CAD build for the part. Positions are in the model's coordinates, mm. A direction names the side the tool comes from. Give positions to 0.01 mm unless a question says otherwise; leave off trailing zeros. Write each loop counter-clockwise with the first axis right and the second up, starting at its lowest first coordinate (ties: lowest second). Pieces come first, ordered by that corner, then holes. Notation, with made-up numbers: (43.25, 88.5) -> (50.25, 88.5) arc R18 cw to (50.25, 116.5) -> close; hole circle Ø4 at (-26.5, 47). An arc over 180 degrees is marked (long way). Answer in a Markdown table with one row per item. Add a question column.
```python
from build123d import *

# Parameters (mm, degrees)
SKETCH008_W          = 9.417664
SKETCH008_H          = 8.015827
PAD_DEPTH            = 6
SKETCH007_W          = 17.214357
SKETCH007_H          = 23
PAD001_DEPTH         = 4
SKETCH_W             = 41
SKETCH_H             = 23
PAD002_DEPTH         = 3
SKETCH009_W          = 6
SKETCH009_H          = 8
PAD003_DEPTH         = 4
POCKET_DEPTH         = 1.5
POCKET001_DEPTH      = 5
POCKET002_DEPTH      = 5
POCKET003_DEPTH      = 5
POCKET004_DEPTH      = 5
SKETCH004_R          = 2.5
POCKET005_DEPTH      = 5
SKETCH010_W          = 41
SKETCH010_H          = 2
SKETCH010_W_2        = 31.58
POCKET006_DEPTH      = 5
SKETCH013_W          = 2
SKETCH013_H          = 2.18
POCKET007_DEPTH      = 10
SKETCH014_W          = 2.7
SKETCH014_H          = 5
POCKET008_DEPTH      = 10
POCKET008_DEPTH_BACK = 10
SKETCH015_W          = 1
SKETCH015_H          = 2.1
POCKET009_DEPTH      = 8.05
SKETCH012_R          = 0.8
POCKET010_DEPTH      = 8
SKETCH016_R          = 0.5
POCKET011_DEPTH      = 1
SKETCH017_W          = 38
SKETCH017_H          = 20
SKETCH017_W_2        = 35
SKETCH017_H_2        = 17
POCKET012_DEPTH      = 0.5


with BuildPart() as part:
    # Sketch008 → Pad (new body)
    with BuildSketch(Plane.XY):
        with Locations((36.336342, 4.0079135)):
            Rectangle(SKETCH008_W, SKETCH008_H)
    extrude(amount=PAD_DEPTH)

    # Sketch007 → Pad001 (join)
    with BuildSketch(Plane.XY):
        with Locations((32.3928215, 11.5)):
            Rectangle(SKETCH007_W, SKETCH007_H)
    extrude(amount=PAD001_DEPTH)

    # Sketch → Pad002 (join)
    with BuildSketch(Plane.XY):
        with Locations((20.5, 11.5)):
            Rectangle(SKETCH_W, SKETCH_H)
    extrude(amount=PAD002_DEPTH)

    # Sketch009 → Pad003 (join)
    with BuildSketch(Plane.XY):
        with Locations((3.029941472, 11.1135029832)):
            Rectangle(SKETCH009_W, SKETCH009_H)
    extrude(amount=PAD003_DEPTH)

    # Sketch003 → Pocket (cut)
    with BuildSketch(Plane.XY):
        with BuildLine():
            Line((23.975689, 13.0540965715), (26.8011965151, 13.0540965715))
            ThreePointArc((26.8011965151, 13.0540965715), (27.3647082361, 13.2875107689), (27.5981224335, 13.8510224899))
            Line((27.5981224335, 13.8510224899), (27.5981224335, 14.526678))
            Line((27.5981224335, 14.526678), (30.5981224335, 14.526678))
            Line((30.5981224335, 14.526678), (30.5981224335, 13.2924514667))
            ThreePointArc((27.3597675383, 10.0540965715), (29.6496302446, 11.0025887604), (30.5981224335, 13.2924514667))
            Line((27.3597675383, 10.0540965715), (23.975689, 10.0540965715))
            Line((23.975689, 10.0540965715), (23.975689, 13.0540965715))
        make_face()
    extrude(amount=POCKET_DEPTH, mode=Mode.SUBTRACT)

    # Sketch001 → Pocket001 (cut)
    with BuildSketch(Plane.XY):
        with BuildLine():
            ThreePointArc((6.1032483008, 13.3387395872), (4.7679879703, 11.5907435275), (5.8459964121, 9.6733734082))
            Line((5.8459964121, 9.6733734082), (11.4677626675, 6.8598227367))
            ThreePointArc((11.4677626675, 6.8598227367), (14.6035600083, 5.8212239037), (17.794301339, 6.6762573881))
            Line((17.794301339, 6.6762573881), (23.3375945955, 9.6414256942))
            ThreePointArc((23.3375945955, 9.6414256942), (24.7768585387, 11.4984422833), (23.4574990247, 13.4424797786))
            Line((23.4574990247, 13.4424797786), (17.8173054197, 16.4670815869))
            ThreePointArc((17.8173054197, 16.4670815869), (14.6646196223, 17.3378254465), (11.5461110533, 16.3516576556))
            Line((11.5461110533, 16.3516576556), (6.1032483008, 13.3387395872))
        make_face()
    extrude(amount=POCKET001_DEPTH, mode=Mode.SUBTRACT)

    # Sketch006 → Pocket002 (cut)
    with BuildSketch(Plane.XY.offset(1.5)):
        with BuildLine():
            ThreePointArc((30.093781, 6.846887), (27.593781, 9.346887), (25.093781, 6.846887))
            Line((25.093781, 6.846887), (25.093781, 5.346887))
            ThreePointArc((25.093781, 5.346887), (27.593781, 2.846887), (30.093781, 5.346887))
            Line((30.093781, 6.846887), (30.093781, 5.346887))
        make_face()
    extrude(amount=POCKET002_DEPTH, mode=Mode.SUBTRACT)

    # Sketch005 → Pocket003 (cut)
    with BuildSketch(Plane.XY.offset(1.5)):
        with BuildLine():
            ThreePointArc((31.548714, 10.251081), (34.048714, 7.751081), (36.548714, 10.251081))
            Line((36.548714, 10.251081), (36.548714, 17.751081))
            ThreePointArc((36.548714, 17.751081), (34.048714, 20.251081), (31.548714, 17.751081))
            Line((31.548714, 10.251081), (31.548714, 17.751081))
        make_face()
    extrude(amount=POCKET003_DEPTH, mode=Mode.SUBTRACT)

    # Sketch002 → Pocket004 (cut)
    with BuildSketch(Plane.XY):
        with BuildLine():
            ThreePointArc((28.798038, 18.6125900268), (26.1467217956, 15.9612738224), (28.798038, 13.3099576181))
            Line((28.798038, 13.309957618), (33.4782685239, 13.309957618))
            ThreePointArc((33.4782685239, 13.3099576181), (36.1295847282, 15.9612738224), (33.4782685239, 18.6125900268))
            Line((28.798038, 18.6125900268), (33.4782685239, 18.6125900268))
        make_face()
    extrude(amount=POCKET004_DEPTH, mode=Mode.SUBTRACT)

    # Sketch004 → Pocket005 (cut)
    with BuildSketch(Plane.XY):
        with Locations((34, 10.25)):
            Circle(SKETCH004_R)
    extrude(amount=POCKET005_DEPTH, mode=Mode.SUBTRACT)

    # Sketch010 → Pocket006 (cut)
    with BuildSketch(Plane.XY.offset(1.8)):
        with Locations((20.5, 22)):
            Rectangle(SKETCH010_W, SKETCH010_H)
        with Locations((15.79, 1)):
            Rectangle(SKETCH010_W_2, SKETCH010_H)
    extrude(amount=POCKET006_DEPTH, mode=Mode.SUBTRACT)

    # Sketch013 → Pocket007 (cut)
    with BuildSketch(Plane.YZ.offset(31.58)):
        with Locations((1, 2.89)):
            Rectangle(SKETCH013_W, SKETCH013_H)
    extrude(amount=POCKET007_DEPTH, mode=Mode.SUBTRACT)

    # Sketch014 → Pocket008 (cut, two sides)
    with BuildSketch(Plane(origin=(0, -2.5, 0), x_dir=(1, 0, 0), z_dir=(0, -0.8660254038, 0.5))) as pocket008_sk:
        with Locations((34.35, 8.5)):
            Rectangle(SKETCH014_W, SKETCH014_H)
    extrude(amount=-POCKET008_DEPTH, mode=Mode.SUBTRACT)
    extrude(pocket008_sk.sketch, amount=POCKET008_DEPTH_BACK, mode=Mode.SUBTRACT)

    # Sketch015 → Pocket009 (cut)
    with BuildSketch(Plane.XZ):
        with Locations((38.5, 5.0085653562)):
            Rectangle(SKETCH015_W, SKETCH015_H)
    extrude(amount=-POCKET009_DEPTH, mode=Mode.SUBTRACT)

    # Sketch012 → Pocket010 (cut)
    with BuildSketch(Plane(origin=(5, 0, 0), x_dir=(0, 1, 0), z_dir=(0.9396926208, 0, -0.3420201433))):
        with Locations((11.55, 1)):
            Circle(SKETCH012_R)
    extrude(amount=-POCKET010_DEPTH, mode=Mode.SUBTRACT)

    # Sketch016 → Pocket011 (cut, symmetric)
    with BuildSketch(Plane(origin=(0, 1, 0.2), x_dir=(1, 0, 0), z_dir=(0, -0.8660254038, 0.5))):
        with Locations((27.497313, 2.982959)):
            Circle(SKETCH016_R)
    extrude(amount=POCKET011_DEPTH, both=True, mode=Mode.SUBTRACT)

    # Sketch017 → Pocket012 (cut)
    with BuildSketch(Plane.XY):
        with Locations((20.5, 11.5)):
            Rectangle(SKETCH017_W, SKETCH017_H)
        with Locations((20.5, 11.5)):
            Rectangle(SKETCH017_W_2, SKETCH017_H_2, mode=Mode.SUBTRACT)
    extrude(amount=POCKET012_DEPTH, mode=Mode.SUBTRACT)


solid = part.part
```
Item 1: Which spindle directions (+Z, -Z, +X, -X, +Y, -Y) get a long thin tool onto all of the face, cutting with end or side? Do faces 1 (the face through (20.68, 14.93, 1.48)), 2 (the face through (38.5, 5, 3.959)), 3 (the face through (25, 13.054, 1)). Say none if no direction does.
Item 2: Slice it at B-B, the plane z = 4.5. List the corners of the cut face in (x, y), then the cut area to 3 significant figures.
Item 3: Mould opens along Y. For faces 4 (the face through (40, 0, 5)), 5 (the face through (39, 4, 5)), 6 (the face through (20.53, 8.14, 1.48)) say: released by +Y, released by -Y, zero draft, split by the parting line, or undercut.
Item 4: Slice it at C-C, the plane x = 34. List the corners of the cut face in (y, z).
Item 5: Slice it at A-A, the plane x = 14. List the corners of the cut face in (y, z).
Item 6: Probe L1, parallel to X at y = 10.25, z = 1.75; L2, parallel to X at y = 16.25, z = 1; L3, parallel to Z at x = 7, y = 15.5. List the from-to ranges inside material, lowest first. Write a range as from..to.
Item 7: Slice it at D-D, the plane y = 19.5. List the corners of the cut face in (x, z).
Item 8: Drop flat-ended pins along their axis: pin 1 Ø1 at (x, z) = (31.5, 3) entering from +Y; pin 2 Ø0.8 at (x, y) = (38.5, 4) entering from +Z; pin 3 Ø1 at (y, z) = (16.5, 5.5) entering from +X; pin 4 Ø1 at (x, z) = (32.5, 5) entering from +Y. Give the stop position or say it passes through.
Answer key:
| question | item | result |
|---|---|---|
| 1 | face 1 | +Z, -Z |
| 1 | face 2 | +Z, -Y |
| 1 | face 3 | -Z |
| 2 | outline | (31.63, 0) -> (38, 0) -> (38, 8.02) -> (35.7, 8.02) -> (35.7, 1.71) -> (33, 1.71) -> (33, 7.96) arc R2.5 cw to (32.88, 8.02) -> (31.63, 8.02) -> close; (39, 0) -> (41.05, 0) -> (41.05, 8.02) -> (39, 8.02) -> close |
| 2 | area | 50.4 mm² |
| 3 | face 4 | released by -Y |
| 3 | face 5 | zero draft |
| 3 | face 6 | undercut |
| 4 | outline | (0, 0) -> (1.5, 0) -> (1.5, 0.5) -> (3, 0.5) -> (3, 0) -> (7.75, 0) -> (7.75, 1.01) -> (0, 5.48) -> (0, 3.98) -> (2, 3.98) -> (2, 1.8) -> (0, 1.8) -> close; (12.75, 0) -> (13.36, 0) -> (13.36, 1.5) -> (12.75, 1.5) -> close; (18.56, 0) -> (20, 0) -> (20, 0.5) -> (21.5, 0.5) -> (21.5, 0) -> (23, 0) -> (23, 1.8) -> (21, 1.8) -> (21, 4) -> (20.25, 4) -> (20.25, 1.5) -> (18.56, 1.5) -> close |
| 5 | outline | (0, 0) -> (1.5, 0) -> (1.5, 0.5) -> (3, 0.5) -> (3, 0) -> (5.87, 0) -> (5.87, 3) -> (2, 3) -> (2, 1.8) -> (0, 1.8) -> close; (17.29, 0) -> (20, 0) -> (20, 0.5) -> (21.5, 0.5) -> (21.5, 0) -> (23, 0) -> (23, 1.8) -> (21, 1.8) -> (21, 3) -> (17.29, 3) -> close |
| 6 | L1 | x = 0..5.16, 24.29..31.5, 36.55..41 |
| 6 | L2 | x = 0..11.36, 18.22..26.16, 36.11..41 |
| 6 | L3 | z = 0..3 |
| 7 | outline | (0, 0) -> (1.5, 0) -> (1.5, 0.5) -> (3, 0.5) -> (3, 0) -> (38, 0) -> (38, 0.5) -> (39.5, 0.5) -> (39.5, 0) -> (41, 0) -> (41, 4) -> (35.84, 4) -> (35.84, 1.5) -> (32.26, 1.5) -> (32.26, 4) -> (23.79, 4) -> (23.79, 3) -> (0, 3) -> close |
| 8 | pin 1 | stops at y = 21 |
| 8 | pin 2 | stops at z = 3.96 |
| 8 | pin 3 | passes through |
| 8 | pin 4 | stops at y = 8.02 |
